Geometry: final body of the model. Coordinates: model frame, mm. A direction names the side the tool comes from. Round coordinates to 2 decimals unless told otherwise and drop trailing zeros. Order: outer loops, then holes, each group sorted by start corner. A loop starts at its lowest first (then second) coordinate and runs counter-clockwise, first axis right, second up. Notation, with made-up numbers: M -19,29 L 27,29 A36 ccw 27,64 Z; hole C -24,-33.5 d9. An arc over 180 degrees is marked long. Put each result on its own line as item: value. Start each with the question number.
1) Section B-B, the plane z = 4. Return loops of the section in (x, y).
2) Section C-C, the plane x = 6.5. Return loops of the section in (y, z).
3) Section D-D, the plane z = 34. Return loops of the section in (x, y).
4) First-contact query: P1, Ø1.1, axis at y = -1, z = 48.5, coming from the +X side; P2, Ø3, axis at y = 2.5, z = 49, coming from the -X side. Flat tips, straight axial feed; report the tip coordinate or a pass-through.
5) Access query for faces 1 (the flat face through (-1, 0, 46.99)), 2 (the cylindrical face through (61.972, 0.178, 49.351)). Directions: +Z, -Z, +X, -X, +Y, -Y. A direction counts if a zero-diameter tool reaches every point of the face in a straight line with its end or side. Return the directions, or none.
6) Material intervals for probe 1 along Y at (x, z) = (16.5, 47.5); probe 2 along X at (y, z) = (-0.5, 5); probe 3 along X at (y, z) = (-0.25, 32), sorted ascending. Write a range as [from, to].
7) Section A-A, the plane y = 8.5. Return loops of the section in (x, z), then the cut area to 3 significant figures.
from build123d import *

# Parameters (mm, degrees)
F0_W     = 127
F0_H     = 25.4
F1_DEPTH = 50.8
F2_W     = 101.6635
F2_H     = 11.4935
F3_DEPTH = 3.81
F5_DEPTH = 50.8
F6_R     = 5.08


with BuildPart() as f1:
    # F0 (on Top) → F1 (new body)
    with BuildSketch(Plane.XY):
        Rectangle(F0_W, F0_H)
    extrude(amount=F1_DEPTH)

    # F2 (on face) → F3 (cut)
    with BuildSketch(Plane.XY.offset(50.8)):
        Rectangle(F2_W, F2_H)
    extrude(amount=-F3_DEPTH, mode=Mode.SUBTRACT)

    # F4 (on face) → F5 (cut)
    with BuildSketch(Plane.XZ.offset(12.7)):
        with BuildLine():
            Line((-57.15, 0), (57.15, 0))
            ThreePointArc((57.15, 0), (0, 41.91), (-57.15, 0))
        make_face()
    extrude(amount=-F5_DEPTH, mode=Mode.SUBTRACT)

    # F6
    f6_edges = [f1.edges().sort_by_distance(p)[0] for p in [
        (-63.5, 0, 50.8),
        (63.5, 0, 50.8),
    ]]
    fillet(f6_edges, radius=F6_R)


solid = f1.part
Result sheet:
1. outline: M -63.5,-12.7 L -55.73,-12.7 L -55.73,12.7 L -63.5,12.7 Z; M 55.73,-12.7 L 63.5,-12.7 L 63.5,12.7 L 55.73,12.7 Z
2. outline: M -12.7,41.56 L 12.7,41.56 L 12.7,50.8 L 5.75,50.8 L 5.75,46.99 L -5.75,46.99 L -5.75,50.8 L -12.7,50.8 Z
3. outline: M -63.5,-12.7 L -29.76,-12.7 L -29.76,12.7 L -63.5,12.7 Z; M 29.76,-12.7 L 63.5,-12.7 L 63.5,12.7 L 29.76,12.7 Z
4. P1: stops at x = 62.98
4. P2: stops at x = -63.18
5. face 1: +Z
5. face 2: +Z, +X, +Y, -Y
6. probe 1: y = [-12.7, -5.75], [5.75, 12.7]
6. probe 2: x = [-63.5, -55.33], [55.33, 63.5]
6. probe 3: x = [-63.5, -33.01], [33.01, 63.5]
7. outline: M -63.5,0 L -57.15,0 A59.92 cw 57.15,0 L 63.5,0 L 63.5,45.72 A5.08 ccw 58.42,50.8 L -58.42,50.8 A5.08 ccw -63.5,45.72 Z
7. area: 2,930 mm2
